```python
from build123d import *

# Parameters (mm, degrees)
EXTRUDE_1_DEPTH     = 7.5
SKETCH_2_R          = 10
CUT_EXTRUDE_1_DEPTH = 111.933538662
SKETCH_3_W          = 2.5
SKETCH_3_H          = 45
CUT_EXTRUDE_2_DEPTH = 111.933538662
FILLET_1_R          = 5
SKETCH_4_R          = 4.25
CUT_EXTRUDE_3_DEPTH = 16.25
M8X1_25_1_D         = 6.8
SKETCH_10_R         = 7
CUT_EXTRUDE_4_DEPTH = 111.933538662
SKETCH_11_W         = 50
SKETCH_11_H         = 50
CUT_EXTRUDE_5_DEPTH = 5
CHAMFER_2_SIZE      = 5
CHAMFER_3_SIZE      = 20
SKETCH_12_R         = 7.25
CUT_EXTRUDE_6_DEPTH = 111.368700273


with BuildPart() as part:
    # 草图1 → 凸台-拉伸1 (new, symmetric)
    with BuildSketch(Plane.XY):
        Polygon((-17.5, 105), (-17.5, 0), (17.5, 0), (17.5, 58), (32.5, 58), (32.5, 105), align=None)
    extrude(amount=EXTRUDE_1_DEPTH, both=True)

    # 草图2 → 切除-拉伸1 (cut, through all)
    with BuildSketch(Plane.XY.offset(7.5)):
        with Locations((0, 30)):
            Circle(SKETCH_2_R)
    extrude(amount=-CUT_EXTRUDE_1_DEPTH, mode=Mode.SUBTRACT)

    # 草图3 → 切除-拉伸2 (cut, through all)
    with BuildSketch(Plane.XY.offset(7.5)):
        with Locations((0, 22.5)):
            Rectangle(SKETCH_3_W, SKETCH_3_H)
    extrude(amount=-CUT_EXTRUDE_2_DEPTH, mode=Mode.SUBTRACT)

    # 圆角1
    fillet_1_edges = [part.edges().sort_by_distance(p)[0] for p in [
        (17.5, 58, 0),
    ]]
    fillet(fillet_1_edges, radius=FILLET_1_R)

    # 草图4 → 切除-拉伸3 (cut)
    with BuildSketch(Plane(origin=(-17.5, 0, 0), x_dir=(0, 0, -1), z_dir=(1, 0, 0))):
        with Locations(Location((0, 8, 0), (0, 0, 270))):
            Circle(SKETCH_4_R)
    extrude(amount=CUT_EXTRUDE_3_DEPTH, mode=Mode.SUBTRACT)

    # M8x1.25 螺纹孔1 (through all)
    with Locations(Plane(origin=(17.5, 13.24526089, -0.849289526), x_dir=(0, 0, -1), z_dir=(1, 0, 0))):
        with Locations((-0.849289526, -5.24526089)):
            Hole(M8X1_25_1_D / 2)

    # 草图10 → 切除-拉伸4 (cut, through all)
    with BuildSketch(Plane.XY.offset(7.5)):
        with Locations((18, 93)):
            Circle(SKETCH_10_R)
    extrude(amount=-CUT_EXTRUDE_4_DEPTH, mode=Mode.SUBTRACT)

    # 草图11 → 切除-拉伸5 (cut)
    with BuildSketch(Plane(origin=(0, 0, -7.5), x_dir=(-1, 0, 0), z_dir=(0, 0, -1))):
        with Locations((-7.5, 80)):
            Rectangle(SKETCH_11_W, SKETCH_11_H)
    extrude(amount=-CUT_EXTRUDE_5_DEPTH, mode=Mode.SUBTRACT)

    # 倒角2
    chamfer_2_edges = [part.edges().sort_by_distance(p)[0] for p in [
        (32.5, 105, 2.5),
        (32.5, 58, 2.5),
    ]]
    chamfer(chamfer_2_edges, length=CHAMFER_2_SIZE)

    # 倒角3
    chamfer_3_edges = [part.edges().sort_by_distance(p)[0] for p in [
        (-17.5, 105, 2.5),
    ]]
    chamfer(chamfer_3_edges, length=CHAMFER_3_SIZE)

    # 草图12 → 切除-拉伸6 (cut, through all)
    with BuildSketch(Plane(origin=(0, 0, -2.5), x_dir=(-1, 0, 0), z_dir=(0, 0, -1))):
        with Locations((-18, 68)):
            Circle(SKETCH_12_R)
    extrude(amount=-CUT_EXTRUDE_6_DEPTH, mode=Mode.SUBTRACT)


solid = part.part
```
Can you work these out from the model? Positions are in its coordinate system, mm. A direction names the side the tool comes from. Coordinates: 2 decimals unless noted, no trailing zeros. Loops run counter-clockwise (first coordinate to the right, second up) from the corner with the lowest first, then second, coordinate; pieces in that order, holes last.
Item 1: Suppose I cut it at C-C (x = 9). Please give me the cut outline in (y, z), then the cut area to 3 significant figures.
Answers below:
outline: (0, -7.5) - (25.64, -7.5) - (25.64, 7.5) - (0, 7.5) - close; (34.36, -7.5) - (55, -7.5) - (55, -2.5) - (105, -2.5) - (105, 7.5) - (34.36, 7.5) - close; hole circle Ø6.8 at (8, 0)
area: 1,160 mm2
Item 2: Please list where these lines run through material, in increasing order: L1, parallel to Y at x = 16, z = 0; L2, parallel to Y at x = 22, z = 2.5; L3, parallel to Y at x = 18, z = 1.5.
Answers below:
L1: y = 0 to 4.6, 11.4 to 61.03, 74.97 to 86.29, 99.71 to 105
L2: y = 57.97 to 61.95, 74.05 to 87.26, 98.74 to 105
L3: y = 55.18 to 60.75, 75.25 to 86, 100 to 105
Item 3: Suppose I cut it at B-B (z = 0). Please give me the cut outline in (x, y).
Answers below:
outline: (-17.5, 0) - (-1.25, 0) - (-1.25, 3.75) - (-17.5, 3.75) - close; (-17.5, 12.25) - (-1.25, 12.25) - (-1.25, 20.08) arc R10 cw to (-1.25, 39.92) - (-1.25, 45) - (1.25, 45) - (1.25, 39.92) arc R10 cw to (1.25, 20.08) - (1.25, 11.4) - (17.5, 11.4) - (17.5, 53) arc R5 cw to (22.5, 58) - (27.5, 58) - (32.5, 63) - (32.5, 100) - (27.5, 105) - (2.5, 105) - (-17.5, 85) - close; (1.25, 0) - (17.5, 0) - (17.5, 4.6) - (1.25, 4.6) - close; hole circle Ø14.5 at (18, 68); hole circle Ø14 at (18, 93)
Item 4: Which directions (+Z, -Z, +X, -X, +Y, -Y) give clear straight access to the entire face, cutting with the end or side of a thin tool? Please do faces 1 (the face through (25, 58, 3)), 2 (the face through (1.25, 42, 0)), 3 (the face through (10, 30, 0)).
Answers below:
face 1: +Z, -Z, +X, -Y
face 2: +Z, -Z, -Y
face 3: +Z, -Z
Item 5: Suppose I cut it at D-D (y = 8). Please give me the cut outline in (x, z), then the cut area to 3 significant figures.
Answers below:
outline: (-17.5, -7.5) - (-1.25, -7.5) - (-1.25, -4.25) - (-17.5, -4.25) - close; (-17.5, 4.25) - (-1.25, 4.25) - (-1.25, 7.5) - (-17.5, 7.5) - close; (1.25, -7.5) - (17.5, -7.5) - (17.5, -3.4) - (1.25, -3.4) - close; (1.25, 3.4) - (17.5, 3.4) - (17.5, 7.5) - (1.25, 7.5) - close
area: 239 mm2
Item 6: Suppose I cut it at A-A (y = 93). Please give me the cut outline in (x, z).
Answers below:
outline: (-9.5, -2.5) - (11, -2.5) - (11, 7.5) - (-9.5, 7.5) - close; (25, -2.5) - (32.5, -2.5) - (32.5, 7.5) - (25, 7.5) - close
Item 7: I'm going to push flat-ended pins straight in: pin 1 (4 mm diameter, centred on x = -5.5, z = -5.5, fed in from +Y); pin 2 (4 mm diameter, centred on y = 43, z = -3, fed in from +X); pin 3 (2.5 mm diameter, centred on x = 26, z = 3, fed in from -Y). Where does each tip first touch, or does it pass through?
Answers below:
pin 1: stops at y = 55
pin 2: stops at x = 17.5
pin 3: stops at y = 58
Item 8: If we mould it in two halves opening along X, with no side actions, what happens to faces 4 (the face through (9, 0, 0)), 5 (the face through (17.09, 99.94, 2.57)), 6 (the face through (32.5, 81, 3))? For each: released by +X, released by -X, zero draft, split by the parting line, or undercut.
Answers below:
face 4: zero draft
face 5: undercut
face 6: released by +X
